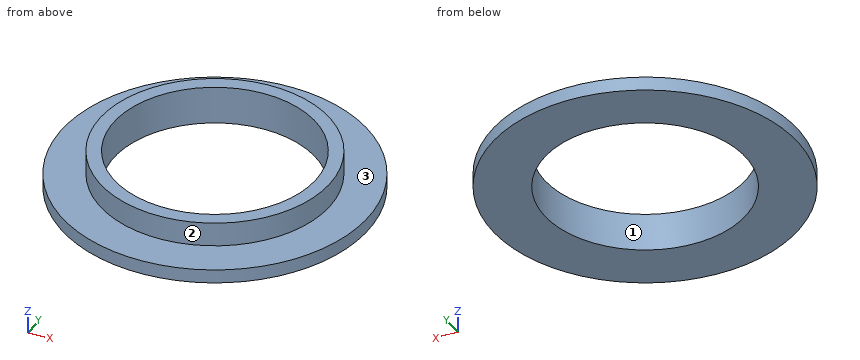
```python
from build123d import *

# Parameters (mm, degrees)
SKETCH1_R               = 44
BOSS_EXTRUDE1_DEPTH     = 4
SKETCH2_R               = 33
BOSS_EXTRUDE2_DEPTH     = 7
SKETCH3_R               = 29
CUT_EXTRUDE1_DEPTH      = 1
CUT_EXTRUDE1_DEPTH_BACK = 12


with BuildPart() as part:
    # Sketch1 → Boss-Extrude1 (new body)
    with BuildSketch(Plane(origin=(0, 0, 0), x_dir=(0, 1, 0), z_dir=(0, 0, 1))):
        Circle(SKETCH1_R)
    extrude(amount=BOSS_EXTRUDE1_DEPTH)

    # Sketch2 → Boss-Extrude2 (add)
    with BuildSketch(Plane.XY.offset(4)):
        Circle(SKETCH2_R)
    extrude(amount=BOSS_EXTRUDE2_DEPTH)

    # Sketch3 → Cut-Extrude1 (cut, two sides)
    with BuildSketch(Plane.XY.offset(11)) as cut_extrude1_sk:
        Circle(SKETCH3_R)
    extrude(amount=CUT_EXTRUDE1_DEPTH, mode=Mode.SUBTRACT)
    extrude(cut_extrude1_sk.sketch, amount=-CUT_EXTRUDE1_DEPTH_BACK, mode=Mode.SUBTRACT)


solid = part.part
```
Work out the finished part from the listing and answer in its coordinate system (mm). Face numbers are marked on the shaded views. Give positions to 0.01 mm unless a question says otherwise; leave off trailing zeros. Write each loop counter-clockwise with the first axis right and the second up, starting at its lowest first coordinate (ties: lowest second). Pieces come first, ordered by that corner, then holes.
(1) Flat-ended cylindrical pins translate along their axes: pin 1 Ø3 at (y, z) = (11, 9) entering from +X; pin 2 Ø8 at (x, y) = (10.5, 18.5) entering from -Z; pin 3 Ø5 at (x, z) = (-12.5, 9.5) entering from +Y; pin 4 Ø2 at (x, z) = (19.5, 8.5) entering from -Y. Find the tip coordinate at first contact, or state that the pin passes through.
Final values:
pin 1: stops at x = 31.6
pin 2: passes through
pin 3: stops at y = 31.45
pin 4: stops at y = -27.33
(2) The part is cut by section D-D on x = 30.5. Write down the section's boundary in (y, z), plus the area to 3 significant figures.
Final values:
outline: (-31.71, 0) - (31.71, 0) - (31.71, 4) - (12.6, 4) - (12.6, 11) - (-12.6, 11) - (-12.6, 4) - (-31.71, 4) - close
area: 430 mm2
(3) Straight lines are drawn through the part: line 1 (Y direction, x = 0, z = 6); line 2 (Y direction, x = 0, z = 0.5). For each, find the intervals that lie inside material, in ascending order.
Final values:
line 1: y = -33 to -29, 29 to 33
line 2: y = -44 to -29, 29 to 44
(4) The part is cut by section C-C on z = 6.25. Write down the section's boundary in (x, y), plus the area to 3 significant figures.
Final values:
outline: circle Ø66 at (0, 0); hole circle Ø58 at (0, 0)
area: 779 mm2
(5) The part is cut by section A-A on x = 0. Write down the section's boundary in (y, z).
Final values:
outline: (-44, 0) - (-29, 0) - (-29, 11) - (-33, 11) - (-33, 4) - (-44, 4) - close; (29, 0) - (44, 0) - (44, 4) - (33, 4) - (33, 11) - (29, 11) - close
(6) The mould has two halves that part along Y. Classify the marked faces 1, 2 and 3: pulls with the +Y half, pulls with the -Y half, needs draft (parallel to the pull), parting line crosses it, or undercut.
Final values:
face 1: undercut
face 2: parting line crosses it
face 3: needs draft
